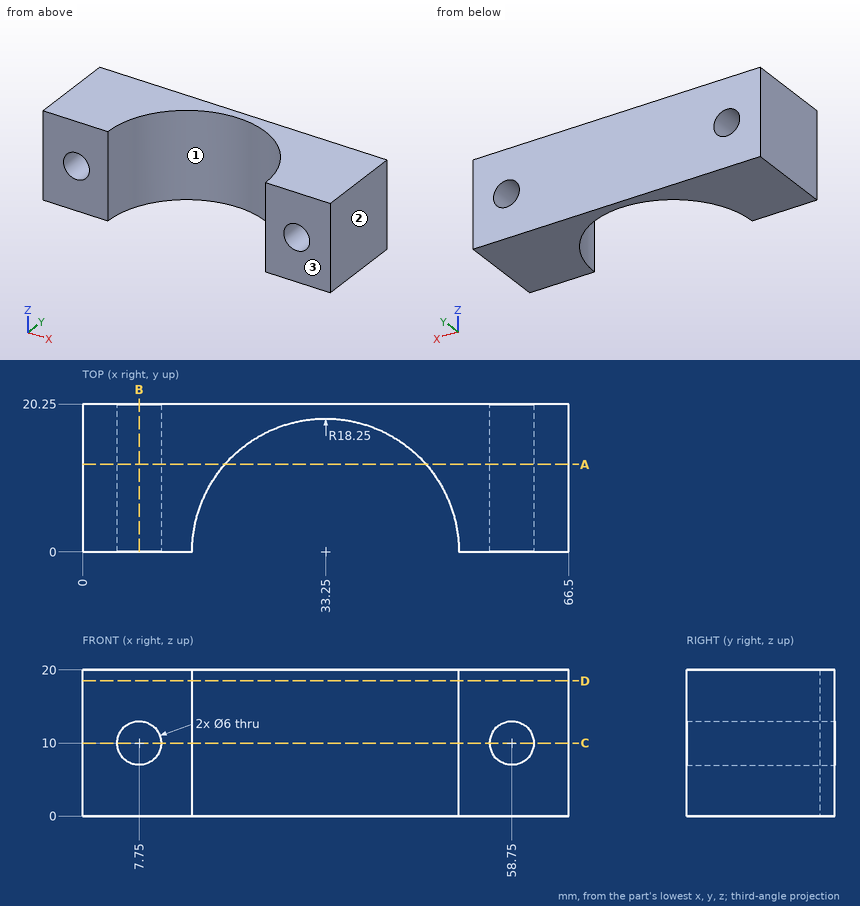
Part print with two shaded views. Sizes in mm from the minimum x, y, z corner. Give positions to 0.01 mm unless a question says otherwise; leave off trailing zeros. Loops run counter-clockwise (first coordinate to the right, second up) from the corner with the lowest first, then second, coordinate; pieces in that order, holes last. Notation, with made-up numbers: (34, -12.75) -> (82, -12.75) arc R35 cw to (82, 23.25) -> close; hole circle Ø7 at (56, 59). An arc over 180 degrees is marked (long way). One line per question, with ' | ' between items.
Q1. Pull direction X, two halves, no side cores. Call the marked faces 1, 2 and 3: pulls with the +X half, pulls with the -X half, needs draft (parallel to the pull), parting line crosses it, or undercut.
Filled sheet:
face 1: undercut | face 2: pulls with the +X half | face 3: needs draft
Q2. Cut at D-D, the plane z = 18.5. Write the cut outline in (x, y).
Filled sheet:
outline: (0, 0) -> (15, 0) arc R18.25 cw to (51.5, 0) -> (66.5, 0) -> (66.5, 20.25) -> (0, 20.25) -> close
Q3. Drill centre lines: line 1 along Z through (x, y) = (7.75, 10.25); line 2 along X through (y, z) = (16, 10); line 3 along X through (y, z) = (8.75, 10). Where is each one in solid material? Low to high. Write a range as [from, to].
Filled sheet:
line 1: z = [0, 7], [13, 20] | line 2: x = [0, 4.75], [10.75, 24.47], [42.03, 55.75], [61.75, 66.5] | line 3: x = [0, 4.75], [10.75, 17.23], [49.27, 55.75], [61.75, 66.5]
Q4. Cut at B-B, the plane x = 7.75. Write the cut outline in (y, z), plus the area to 4 significant figures.
Filled sheet:
outline: (0, 0) -> (20.25, 0) -> (20.25, 7) -> (0, 7) -> close; (0, 13) -> (20.25, 13) -> (20.25, 20) -> (0, 20) -> close | area: 283.5 mm²
Q5. Cut at C-C, the plane z = 10. Write the cut outline in (x, y), plus the area to 3 significant figures.
Filled sheet:
outline: (0, 0) -> (4.75, 0) -> (4.75, 20.25) -> (0, 20.25) -> close; (10.75, 0) -> (15, 0) arc R18.25 cw to (51.5, 0) -> (55.75, 0) -> (55.75, 20.25) -> (10.75, 20.25) -> close; (61.75, 0) -> (66.5, 0) -> (66.5, 20.25) -> (61.75, 20.25) -> close | area: 580 mm²
Q6. Drop flat-ended pins along their axis: pin 1 (12 mm diameter, centred on x = 29.5, z = 16, fed in from -Y); pin 2 (4 mm diameter, centred on x = 31, z = 3, fed in from -Y). Give the stop position or say it passes through.
Filled sheet:
pin 1: stops at y = 15.43 | pin 2: stops at y = 17.75
Q7. Cut at A-A, the plane y = 12. Write the cut outline in (x, z).
Filled sheet:
outline: (0, 0) -> (19.5, 0) -> (19.5, 20) -> (0, 20) -> close; (47, 0) -> (66.5, 0) -> (66.5, 20) -> (47, 20) -> close; hole circle Ø6 at (7.75, 10); hole circle Ø6 at (58.75, 10)
